Check sheet for the modelled part. Datum: model origin and axes. Units: mm. Round coordinates to 2 decimals unless told otherwise and drop trailing zeros. Loops run counter-clockwise (first coordinate to the right, second up) from the corner with the lowest first, then second, coordinate; pieces in that order, holes last. Notation, with made-up numbers: (-13, -36) - (32, -36) arc R11 cw to (32, -15) - close; hole circle Ø10 at (89, 54). An arc over 180 degrees is marked (long way). Put each result on its own line as item: value. Start each with the question number.
Item 1: Material ranges on line 1 along Z through (x, y) = (-12, -16.25); line 2 along Z through (x, y) = (78.5, -4.25), recorded low to high.
Item 2: Section check A-A, the plane y = -20.5. Record the cut outline in (x, z).
Item 3: Section check C-C, the plane x = 56.5. Record the cut outline in (y, z), and give its area (3 significant figures).
Item 4: Gauge pin test, flat ends, axial feed: pin 1 Ø6 at (x, y) = (60, -5) entering from -Z; pin 2 Ø1 at (x, z) = (35.5, -54.5) entering from +Y; pin 3 Ø10 at (x, y) = (32, -14.5) entering from -Z. Record the tip position at first contact, or that the pin passes through.
Item 5: Section check B-B, the plane x = 82. Record the cut outline in (y, z), and give its area (3 significant figures).
from build123d import *

# Parameters (mm, degrees)
F0_W     = 123.1974195689
F0_H     = 95.799991861
F1_DEPTH = 23.368


with BuildPart() as f1:
    # F0 (on Front) → F1 (new body)
    with BuildSketch(Plane.XZ):
        Polygon((113.2330745459, -4.5672673732), (106.6863015294, -9.379176423), (106.6863015294, -105.1791682839), (113.2330745459, -105.1791682839), align=None)
        Polygon((-16.5111180395, -9.379176423), (106.6863015294, -9.379176423), (113.2330745459, -4.5672673732), (-16.5111180395, -4.5672673732), align=None)
        Polygon((-16.5111180395, -105.1791682839), (-16.5111180395, -9.379176423), (-22.6063877344, -9.379176423), (-22.6063877344, -101.0192483664), (-22.6063877344, -113.7807220221), align=None)
        Polygon((-22.6063877344, -9.379176423), (-16.5111180395, -9.379176423), (-16.5111180395, -4.5672673732), align=None)
        Polygon((113.2330745459, -105.1791682839), (106.6863015294, -105.1791682839), (106.6863015294, -110.7390969992), align=None)
        Polygon((106.6863015294, -110.7390969992), (106.6863015294, -105.1791682839), (-16.5111180395, -105.1791682839), (-22.6063877344, -113.7807220221), align=None)
        with Locations((45.087591745, -57.2791723534)):
            Rectangle(F0_W, F0_H)
    extrude(amount=F1_DEPTH)


solid = f1.part
Check result:
1. line 1: -113.53 to -4.57
1. line 2: -111.4 to -4.57
2. outline: (-22.61, -113.78) - (106.69, -110.74) - (113.23, -105.18) - (113.23, -4.57) - (-16.51, -4.57) - (-22.61, -9.38) - close
3. outline: (-23.37, -111.92) - (0, -111.92) - (0, -4.57) - (-23.37, -4.57) - close
3. area: 2,510 mm²
4. pin 1: z = -111.91
4. pin 2: y = 0
4. pin 3: z = -112.61
5. outline: (-23.37, -111.32) - (0, -111.32) - (0, -4.57) - (-23.37, -4.57) - close
5. area: 2,490 mm²
